For this review, take the finished solid that the model builds, in its own axes (mm). Face numbers are marked on the shaded views. A direction names the side the tool comes from. Round coordinates to 2 decimals unless told otherwise and drop trailing zeros. Order: outer loops, then holes, each group sorted by start corner. A loop starts at its lowest first (then second) coordinate and runs counter-clockwise, first axis right, second up. Notation, with made-up numbers: M -25,32 L -17,32 A13 cw -17,49 Z; hole C -34,44.5 d10. An arc over 180 degrees is marked long. Write item = value, one per line. Start each with the question number.
from build123d import *

# Parameters (mm, degrees)
F0_R     = 42.5
F0_R_2   = 4
F0_R_3   = 12.5
F1_DEPTH = 6
F2_R     = 17.5
F2_R_2   = 12.5
F3_DEPTH = 10


with BuildPart() as f1:
    # F0 (on Top) → F1 (new body)
    with BuildSketch(Plane.XY):
        Circle(F0_R)
        with Locations((0, -28.630458)):
            Circle(F0_R_2, mode=Mode.SUBTRACT)
        with Locations((-28.630458, 0)):
            Circle(F0_R_2, mode=Mode.SUBTRACT)
        Circle(F0_R_3, mode=Mode.SUBTRACT)
        with Locations((28.630458, 0)):
            Circle(F0_R_2, mode=Mode.SUBTRACT)
        with Locations((0, 28.630458)):
            Circle(F0_R_2, mode=Mode.SUBTRACT)
    extrude(amount=F1_DEPTH)

    # F2 (on face) → F3 (join)
    with BuildSketch(Plane.XY.offset(6)):
        Circle(F2_R)
        Circle(F2_R_2, mode=Mode.SUBTRACT)
    extrude(amount=F3_DEPTH)


solid = f1.part
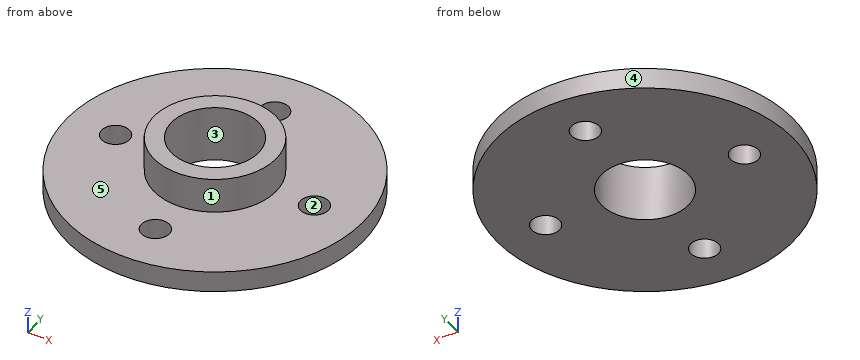
(1) Draft analysis for pull direction X (two halves, no side actions). For the marked faces 3, 4 and 5, state which applies: released by +X, released by -X, zero draft, split by the parting line, or undercut.
(2) For line 1 along Y through (x, z) = (0, 1.4); line 2 along Y through (x, z) = (0, 11); line 3 along Z through (x, y) = (-30, -13.5), list the stretches that pass through material, from the lowest coordinate up.
(3) We need section B-B, the plane x = 3. Write out the cut boundary in (y, z).
(4) For the marked faces 1 and 2, list the 3-axis set-ups (+Z, -Z, +X, -X, +Y, -Y) from which the entire face can be reached by the end or side of a thin tool; tool diameter is ignored.
(5) Insertion check: pin 1 (1 mm diameter, centred on x = 6, z = 13.5, fed in from -Y); pin 2 (3 mm diameter, centred on y = 9, z = 2.5, fed in from +X); pin 3 (8 mm diameter, centred on y = 29, z = 2, fed in from +X); pin 4 (1.5 mm diameter, centred on x = -6, y = -28.5, fed in from -Z). Each pin has a flat end and moves straight along its axis. Give the tip position at first contact, or say it passes through.
(6) We need section A-A, the plane y = 0. Write out the cut boundary in (x, z).
(7) We need section C-C, the plane z = 14.25. Write out the cut boundary in (x, y).
(8) We need section D-D, the plane y = -8.5. Write out the cut boundary in (x, z), then the cut area to 3 significant figures.
Values:
q1.face_3 = undercut
q1.face_4 = split by the parting line
q1.face_5 = zero draft
q2.line_1 = -42.5 to -32.63, -24.63 to -12.5, 12.5 to 24.63, 32.63 to 42.5
q2.line_2 = -17.5 to -12.5, 12.5 to 17.5
q2.line_3 = 0 to 6
q3.outline = M -42.39,0 L -31.28,0 L -31.28,6 L -42.39,6 Z; M -25.98,0 L -12.13,0 L -12.13,16 L -17.24,16 L -17.24,6 L -25.98,6 Z; M 12.13,0 L 25.98,0 L 25.98,6 L 17.24,6 L 17.24,16 L 12.13,16 Z; M 31.28,0 L 42.39,0 L 42.39,6 L 31.28,6 Z
q4.face_1 = +Z
q4.face_2 = +Z, -Z
q5.pin_1 = -16.61
q5.pin_2 = 41.83
q5.pin_3 = 34.37
q5.pin_4 = 0
q6.outline = M -42.5,0 L -32.63,0 L -32.63,6 L -42.5,6 Z; M -24.63,0 L -12.5,0 L -12.5,16 L -17.5,16 L -17.5,6 L -24.63,6 Z; M 12.5,0 L 24.63,0 L 24.63,6 L 17.5,6 L 17.5,16 L 12.5,16 Z; M 32.63,0 L 42.5,0 L 42.5,6 L 32.63,6 Z
q7.outline = C 0,0 d35; hole C 0,0 d25
q8.outline = M -41.64,0 L -9.17,0 L -9.17,16 L -15.3,16 L -15.3,6 L -41.64,6 Z; M 9.17,0 L 41.64,0 L 41.64,6 L 15.3,6 L 15.3,16 L 9.17,16 Z
q8.area = 512 mm²
